Work out the finished part from the listing and answer in its coordinate system (mm). A direction names the side the tool comes from. Coordinates: 2 decimals unless noted, no trailing zeros. Order: outer loops, then holes, each group sorted by start corner. A loop starts at its lowest first (then second) coordinate and runs counter-clockwise, first axis right, second up. Notation, with made-up numbers: M -19,-4 L 24,-4 A7 cw 24,8 Z; hole C 67,19 d7. An arc over 180 degrees is marked long. Answer in a Markdown table with one row per item. Add a question column.
Item 1: The part is cut by section B-B (y = 5). State how many separate pieces and enclosed holes the cut face has, then the cut area to 3 significant figures.
Item 2: Consider line 1 (X direction, y = 8.5, z = 83); line 2 (X direction, y = 5, z = 95); line 3 (X direction, y = 5.75, z = 0). Determine where each line is inside the solid, lowest interval first. Write a range as from..to.
Item 3: Flat-ended cylindrical pins translate along their axes: pin 1 Ø4 at (x, y) = (-8.5, 4) entering from -Z; pin 2 Ø5.5 at (x, y) = (7, 3.5) entering from -Z; pin 3 Ø2 at (x, y) = (6.5, 2.5) entering from -Z. Find the tip coordinate at first contact, or state that the pin passes through.
Item 4: The part is cut by section D-D (z = 0). Write down the section's boundary in (x, y).
Item 5: The mould has two halves that part along X. Classify faces 1 (the face through (0, 10, 54)), 2 (the face through (-7, 5, 79.5)), 3 (the face through (15, 5, 50)): released by +X, released by -X, zero draft, split by the parting line, or undercut.
Item 6: The part is cut by section A-A (z = 84). Write down the section's boundary in (x, y).
Item 7: Which of the six approach directions +Z, -Z, +X, -X, +Y, -Y give full straight-line access (tool end or side, diameter ignored) to faces 4 (the face through (1.5, 5, 85)), 5 (the face through (0, 5, 100))?
Item 8: The part is cut by section C-C (x = -2.5). Write down the section's boundary in (y, z).
from build123d import *

# Parameters (mm, degrees)
SKETCH_1_R                  = 12.5
EXTRUDE_1_DEPTH             = 10
CUT_EXTRUDE_5_DEPTH         = 102.687019821
SKETCH_8_W                  = 1.65
SKETCH_8_H                  = 14
HOLE_WIZARD_M41_D           = 4.5
HOLE_WIZARD_M41_DEPTH       = 14
HOLE_WIZARD_M41_CBORE_D     = 8
HOLE_WIZARD_M41_CBORE_DEPTH = 4.5
CUT_EXTRUDE_START           = -10
CUT_EXTRUDE_6_DEPTH         = 10
FILLET_1_R                  = 10
M4X0_72_D                   = 3.3
M4X0_72_DEPTH               = 10
M4X0_72_TIP                 = 0.991420021
CUT_EXTRUDE_7_DEPTH         = 102.612007273
EXTRUDE_2_DEPTH             = 10


with BuildPart() as part:
    # Эскиз1 → Бобышка-Вытянуть1 (new body)
    with BuildSketch(Plane(origin=(0, 0, 0), x_dir=(1, 0, 0), z_dir=(0, 1, 0))):
        with BuildLine():
            Line((-15.5, 0), (-15.5, -100))
            Line((-15.5, -100), (15.5, -100))
            Line((15.5, -100), (15.5, 0))
            ThreePointArc((15.5, 0), (0, 15.5), (-15.5, 0))
        make_face()
        with Locations(Location((0, 0, 0), (0, 0, 270))):
            Circle(SKETCH_1_R, mode=Mode.SUBTRACT)
    extrude(amount=EXTRUDE_1_DEPTH)

    # Эскиз6 → Вырез-Вытянуть5 (cut, through all)
    with BuildSketch(Plane(origin=(0, 10, 0), x_dir=(1, 0, 0), z_dir=(0, 1, 0))):
        with BuildLine():
            Line((-1.5, -12.409673646), (-1.5, -26))
            ThreePointArc((-1.5, -26), (0, -27.5), (1.5, -26))
            Line((1.5, -26), (1.5, -12.409673646))
            ThreePointArc((1.5, -12.409673646), (0, -12.5), (-1.5, -12.409673646))
        make_face()
        with BuildLine():
            Line((-1.5, -42.5), (-1.5, -49.5))
            ThreePointArc((-1.5, -49.5), (-2.085786438, -50.914213562), (-3.5, -51.5))
            Line((-3.5, -51.5), (-10.5, -51.5))
            ThreePointArc((-10.5, -51.5), (-11.914213562, -50.914213562), (-12.5, -49.5))
            Line((-12.5, -49.5), (-12.5, -42.5))
            ThreePointArc((-12.5, -42.5), (-11.914213562, -41.085786438), (-10.5, -40.5))
            Line((-10.5, -40.5), (-3.5, -40.5))
            ThreePointArc((-3.5, -40.5), (-2.085786438, -41.085786438), (-1.5, -42.5))
        make_face()
        with BuildLine():
            Line((-1.5, -55.5), (-1.5, -62.5))
            ThreePointArc((-1.5, -62.5), (-2.085786438, -63.914213562), (-3.5, -64.5))
            Line((-3.5, -64.5), (-10.5, -64.5))
            ThreePointArc((-10.5, -64.5), (-11.914213562, -63.914213562), (-12.5, -62.5))
            Line((-12.5, -62.5), (-12.5, -55.5))
            ThreePointArc((-12.5, -55.5), (-11.914213562, -54.085786438), (-10.5, -53.5))
            Line((-10.5, -53.5), (-3.5, -53.5))
            ThreePointArc((-3.5, -53.5), (-2.085786438, -54.085786438), (-1.5, -55.5))
        make_face()
        with BuildLine():
            Line((-1.5, -68.5), (-1.5, -75.5))
            ThreePointArc((-1.5, -75.5), (-2.085786438, -76.914213562), (-3.5, -77.5))
            Line((-3.5, -77.5), (-10.5, -77.5))
            ThreePointArc((-10.5, -77.5), (-11.914213562, -76.914213562), (-12.5, -75.5))
            Line((-12.5, -75.5), (-12.5, -68.5))
            ThreePointArc((-12.5, -68.5), (-11.914213562, -67.085786438), (-10.5, -66.5))
            Line((-10.5, -66.5), (-3.5, -66.5))
            ThreePointArc((-3.5, -66.5), (-2.085786438, -67.085786438), (-1.5, -68.5))
        make_face()
        with BuildLine():
            Line((-1.5, -81.5), (-1.5, -88.5))
            ThreePointArc((-1.5, -88.5), (-2.085786438, -89.914213562), (-3.5, -90.5))
            Line((-3.5, -90.5), (-10.5, -90.5))
            ThreePointArc((-10.5, -90.5), (-11.914213562, -89.914213562), (-12.5, -88.5))
            Line((-12.5, -88.5), (-12.5, -81.5))
            ThreePointArc((-12.5, -81.5), (-11.914213562, -80.085786438), (-10.5, -79.5))
            Line((-10.5, -79.5), (-3.5, -79.5))
            ThreePointArc((-3.5, -79.5), (-2.085786438, -80.085786438), (-1.5, -81.5))
        make_face()
        with BuildLine():
            Line((1.5, -29.5), (1.5, -36.5))
            ThreePointArc((1.5, -36.5), (2.085786438, -37.914213562), (3.5, -38.5))
            Line((3.5, -38.5), (10.5, -38.5))
            ThreePointArc((10.5, -38.5), (11.914213562, -37.914213562), (12.5, -36.5))
            Line((12.5, -36.5), (12.5, -29.5))
            ThreePointArc((12.5, -29.5), (11.914213562, -28.085786438), (10.5, -27.5))
            Line((10.5, -27.5), (3.5, -27.5))
            ThreePointArc((3.5, -27.5), (2.085786438, -28.085786438), (1.5, -29.5))
        make_face()
        with BuildLine():
            Line((-12.5, -29.5), (-12.5, -36.5))
            ThreePointArc((-12.5, -36.5), (-11.914213562, -37.914213562), (-10.5, -38.5))
            Line((-10.5, -38.5), (-3.5, -38.5))
            ThreePointArc((-3.5, -38.5), (-2.085786438, -37.914213562), (-1.5, -36.5))
            Line((-1.5, -36.5), (-1.5, -29.5))
            ThreePointArc((-1.5, -29.5), (-2.085786438, -28.085786438), (-3.5, -27.5))
            Line((-3.5, -27.5), (-10.5, -27.5))
            ThreePointArc((-10.5, -27.5), (-11.914213562, -28.085786438), (-12.5, -29.5))
        make_face()
        with BuildLine():
            Line((10.5, -79.5), (3.5, -79.5))
            ThreePointArc((3.5, -79.5), (2.085786438, -80.085786438), (1.5, -81.5))
            Line((1.5, -81.5), (1.5, -88.5))
            ThreePointArc((1.5, -88.5), (2.085786438, -89.914213562), (3.5, -90.5))
            Line((3.5, -90.5), (10.5, -90.5))
            ThreePointArc((10.5, -90.5), (11.914213562, -89.914213562), (12.5, -88.5))
            Line((12.5, -88.5), (12.5, -81.5))
            ThreePointArc((12.5, -81.5), (11.914213562, -80.085786438), (10.5, -79.5))
        make_face()
        with BuildLine():
            Line((10.5, -66.5), (3.5, -66.5))
            ThreePointArc((3.5, -66.5), (2.085786438, -67.085786438), (1.5, -68.5))
            Line((1.5, -68.5), (1.5, -75.5))
            ThreePointArc((1.5, -75.5), (2.085786438, -76.914213562), (3.5, -77.5))
            Line((3.5, -77.5), (10.5, -77.5))
            ThreePointArc((10.5, -77.5), (11.914213562, -76.914213562), (12.5, -75.5))
            Line((12.5, -75.5), (12.5, -68.5))
            ThreePointArc((12.5, -68.5), (11.914213562, -67.085786438), (10.5, -66.5))
        make_face()
        with BuildLine():
            Line((10.5, -53.5), (3.5, -53.5))
            ThreePointArc((3.5, -53.5), (2.085786438, -54.085786438), (1.5, -55.5))
            Line((1.5, -55.5), (1.5, -62.5))
            ThreePointArc((1.5, -62.5), (2.085786438, -63.914213562), (3.5, -64.5))
            Line((3.5, -64.5), (10.5, -64.5))
            ThreePointArc((10.5, -64.5), (11.914213562, -63.914213562), (12.5, -62.5))
            Line((12.5, -62.5), (12.5, -55.5))
            ThreePointArc((12.5, -55.5), (11.914213562, -54.085786438), (10.5, -53.5))
        make_face()
        with BuildLine():
            Line((10.5, -40.5), (3.5, -40.5))
            ThreePointArc((3.5, -40.5), (2.085786438, -41.085786438), (1.5, -42.5))
            Line((1.5, -42.5), (1.5, -49.5))
            ThreePointArc((1.5, -49.5), (2.085786438, -50.914213562), (3.5, -51.5))
            Line((3.5, -51.5), (10.5, -51.5))
            ThreePointArc((10.5, -51.5), (11.914213562, -50.914213562), (12.5, -49.5))
            Line((12.5, -49.5), (12.5, -42.5))
            ThreePointArc((12.5, -42.5), (11.914213562, -41.085786438), (10.5, -40.5))
        make_face()
    extrude(amount=-CUT_EXTRUDE_5_DEPTH, mode=Mode.SUBTRACT)

    # Эскиз8 → Отверстие обработанное метчиком M4x0.71 (revolve, cut)
    with BuildSketch(Plane(origin=(1.5, 5, 17.409673646), x_dir=(0, 0, 1), z_dir=(0, 1, 0))):
        with Locations((0.825, 7)):
            Rectangle(SKETCH_8_W, SKETCH_8_H)
    revolve(axis=Axis((-4.85, 5, 17.409673646), (1, 0, 0)), mode=Mode.SUBTRACT)

    # Цековка для винта с внутренним шестигранником M41
    with Locations(Plane.ZY.offset(15.5)):
        with Locations((17.409673646, 5)):
            CounterBoreHole(HOLE_WIZARD_M41_D / 2, HOLE_WIZARD_M41_CBORE_D / 2, HOLE_WIZARD_M41_CBORE_DEPTH, depth=HOLE_WIZARD_M41_DEPTH)

    # Эскиз12 → Вырез-Вытянуть6 (cut)
    with BuildSketch(Plane(origin=(0, 10, 0), x_dir=(1, 0, 0), z_dir=(0, 1, 0)).offset(CUT_EXTRUDE_START)):
        with BuildLine():
            Line((-15, 3.905124838), (-15, -100))
            Line((-15, -100), (-15.5, -100))
            Line((-15.5, -100), (-15.5, 0))
            ThreePointArc((-15.5, 0), (-15.374491862, 1.968501969), (-15, 3.905124838))
        make_face()
        with BuildLine():
            Line((15, -100), (15, 3.905124838))
            ThreePointArc((15, 3.905124838), (15.374491862, 1.968501969), (15.5, 0))
            Line((15.5, 0), (15.5, -100))
            Line((15.5, -100), (15, -100))
        make_face()
    extrude(amount=CUT_EXTRUDE_6_DEPTH, mode=Mode.SUBTRACT)

    # Скругление1
    fillet_1_edges = [part.edges().sort_by_distance(p)[0] for p in [
        (15, 5, -3.905124838),
        (-15, 5, -3.905124838),
    ]]
    fillet(fillet_1_edges, radius=FILLET_1_R)

    # Отверстие обработанное метчиком M4x0.72
    with Locations(Plane.XY.offset(100)):
        with Locations((-9.998288453, 5), (10.001711547, 5)):
            Hole(M4X0_72_D / 2, depth=M4X0_72_DEPTH)
            with Locations((0, 0, -(M4X0_72_DEPTH + M4X0_72_TIP / 2))):  # 118° drill point
                Cone(0, M4X0_72_D / 2, M4X0_72_TIP, mode=Mode.SUBTRACT)

    # Эскиз16 → Вырез-Вытянуть7 (cut, through all)
    with BuildSketch(Plane(origin=(0, 10, 0), x_dir=(1, 0, 0), z_dir=(0, 1, 0))):
        with BuildLine():
            Line((1.5, -26), (1.5, -45))
            ThreePointArc((1.5, -45), (0, -46.5), (-1.5, -45))
            Line((-1.5, -45), (-1.5, -26))
            ThreePointArc((-1.5, -26), (0, -24.5), (1.5, -26))
        make_face()
    extrude(amount=-CUT_EXTRUDE_7_DEPTH, mode=Mode.SUBTRACT)

    # Эскиз17 → Бобышка-Вытянуть2 (add, through all)
    with BuildSketch(Plane(origin=(0, 10, 0), x_dir=(1, 0, 0), z_dir=(0, 1, 0))):
        with BuildLine():
            Line((-1.5, -29.5), (-1.5, -36.5))
            ThreePointArc((-1.5, -36.5), (-2.085786438, -37.914213562), (-3.5, -38.5))
            Line((-3.5, -38.5), (-5.5, -38.5))
            ThreePointArc((-5.5, -38.5), (-4.085786438, -37.914213562), (-3.5, -36.5))
            Line((-3.5, -36.5), (-3.5, -29.5))
            ThreePointArc((-3.5, -29.5), (-4.085786438, -28.085786438), (-5.5, -27.5))
            Line((-5.5, -27.5), (-3.5, -27.5))
            ThreePointArc((-3.5, -27.5), (-2.085786438, -28.085786438), (-1.5, -29.5))
        make_face()
        with BuildLine():
            Line((-1.5, -42.5), (-1.5, -49.5))
            ThreePointArc((-1.5, -49.5), (-2.085786438, -50.914213562), (-3.5, -51.5))
            Line((-3.5, -51.5), (-5.5, -51.5))
            ThreePointArc((-5.5, -51.5), (-4.085786438, -50.914213562), (-3.5, -49.5))
            Line((-3.5, -49.5), (-3.5, -42.5))
            ThreePointArc((-3.5, -42.5), (-4.085786438, -41.085786438), (-5.5, -40.5))
            Line((-5.5, -40.5), (-3.5, -40.5))
            ThreePointArc((-3.5, -40.5), (-2.085786438, -41.085786438), (-1.5, -42.5))
        make_face()
        with BuildLine():
            Line((5.5, -51.5), (3.5, -51.5))
            ThreePointArc((3.5, -51.5), (2.085786438, -50.914213562), (1.5, -49.5))
            Line((1.5, -49.5), (1.5, -42.5))
            ThreePointArc((1.5, -42.5), (2.085786438, -41.085786438), (3.5, -40.5))
            Line((3.5, -40.5), (5.5, -40.5))
            ThreePointArc((5.5, -40.5), (4.085786438, -41.085786438), (3.5, -42.5))
            Line((3.5, -42.5), (3.5, -49.5))
            ThreePointArc((3.5, -49.5), (4.085786438, -50.914213562), (5.5, -51.5))
        make_face()
        with BuildLine():
            Line((5.5, -38.5), (3.5, -38.5))
            ThreePointArc((3.5, -38.5), (2.085786438, -37.914213562), (1.5, -36.5))
            Line((1.5, -36.5), (1.5, -29.5))
            ThreePointArc((1.5, -29.5), (2.085786438, -28.085786438), (3.5, -27.5))
            Line((3.5, -27.5), (5.5, -27.5))
            ThreePointArc((5.5, -27.5), (4.085786438, -28.085786438), (3.5, -29.5))
            Line((3.5, -29.5), (3.5, -36.5))
            ThreePointArc((3.5, -36.5), (4.085786438, -37.914213562), (5.5, -38.5))
        make_face()
    extrude(amount=-EXTRUDE_2_DEPTH)


solid = part.part
Reply:
| question | item | result |
|---|---|---|
| 1 | separate pieces | 2 |
| 1 | enclosed holes | 8 |
| 1 | area | 1,510 mm2 |
| 2 | line 1 | x = -15..-12.5, -1.5..1.5, 12.5..15 |
| 2 | line 2 | x = -15..-11.65, -8.35..8.35, 11.65..15 |
| 2 | line 3 | x = -15..-12.5, 12.5..15 |
| 3 | pin 1 | stops at z = -14.07 |
| 3 | pin 2 | stops at z = -14.91 |
| 3 | pin 3 | stops at z = -14.49 |
| 4 | outline | M -15,0 L -12.5,0 L -12.5,10 L -15,10 Z; M 12.5,0 L 15,0 L 15,10 L 12.5,10 Z |
| 5 | face 1 | zero draft |
| 5 | face 2 | undercut |
| 5 | face 3 | released by +X |
| 6 | outline | M -15,0 L -12.5,0 L -12.5,10 L -15,10 Z; M -1.5,0 L 1.5,0 L 1.5,10 L -1.5,10 Z; M 12.5,0 L 15,0 L 15,10 L 12.5,10 Z |
| 7 | face 4 | +Y, -Y |
| 7 | face 5 | +Z, +X, -X, +Y, -Y |
| 8 | outline | M 0,-15.3 L 10,-15.3 L 10,-12.25 L 0,-12.25 Z; M 0,12.25 L 10,12.25 L 10,53.77 L 0,53.77 Z; M 0,64.23 L 10,64.23 L 10,66.77 L 0,66.77 Z; M 0,77.23 L 10,77.23 L 10,79.77 L 0,79.77 Z; M 0,90.23 L 10,90.23 L 10,100 L 0,100 Z; hole C 5,17.41 d4.5 |
